Could you check a few things on this model? Use its own coordinates, in mm. Face numbers are marked on the shaded views. A direction names the side the tool comes from. Give positions to 0.01 mm unless a question says otherwise; leave off trailing zeros. Write each loop counter-clockwise with the first axis right and the second up, starting at its lowest first coordinate (ties: lowest second). Pieces come first, ordered by that corner, then holes. Notation, with made-up numbers: (-30.75, -8) - (21.25, -8) arc R18 ccw to (21.25, 18) - close; hole circle Ø8 at (-15.5, -27.5). An arc over 180 degrees is marked (long way). Answer in a Markdown table with one row per item.
from build123d import *

# Parameters (mm, degrees)
SKETCH1_R           = 7.338508892
SKETCH1_W           = 14.683745891
SKETCH1_H           = 15.594449323
BOSS_EXTRUDE6_DEPTH = 7.62


with BuildPart() as part:
    # Sketch1 → Boss-Extrude6 (new body)
    with BuildSketch(Plane(origin=(0, 0, 0), x_dir=(1, 0, 0), z_dir=(0, 1, 0))):
        with BuildLine():
            Line((-33.85382456, 51.361208868), (6.15117544, 51.361208868))
            ThreePointArc((6.15117544, 51.361208868), (9.743277889, 49.873311317), (11.23117544, 46.281208868))
            Line((11.23117544, 46.281208868), (11.23117544, 16.055208868))
            ThreePointArc((11.23117544, 16.055208868), (9.743277889, 12.46310642), (6.15117544, 10.975208868))
            Line((6.15117544, 10.975208868), (-33.85382456, 10.975208868))
            ThreePointArc((-33.85382456, 10.975208868), (-37.445927008, 12.46310642), (-38.93382456, 16.055208868))
            Line((-38.93382456, 16.055208868), (-38.93382456, 46.281208868))
            ThreePointArc((-38.93382456, 46.281208868), (-37.445927008, 49.873311317), (-33.85382456, 51.361208868))
        make_face()
        with Locations((-26.728784531, 42.288093859)):
            Circle(SKETCH1_R, mode=Mode.SUBTRACT)
        Polygon((-26.110126673, 13.007611736), (-27.479198511, 18.629319113), (-33.847743068, 18.629319113), (-28.993277919, 22.103725346), (-30.892236597, 27.725432723), (-26.110126673, 24.705324634), (-21.328016749, 27.725432723), (-23.076426813, 22.103725346), (-18.372510278, 18.629319113), (-24.17123819, 18.974896902), align=None, mode=Mode.SUBTRACT)
        with Locations((-1.086674016, 42.41081801)):
            Rectangle(SKETCH1_W, SKETCH1_H, mode=Mode.SUBTRACT)
        Polygon((5.867569864, 19.665294437), (-7.758291576, 27.532189206), (-7.758291576, 11.798399667), align=None, mode=Mode.SUBTRACT)
    extrude(amount=BOSS_EXTRUDE6_DEPTH)


solid = part.part
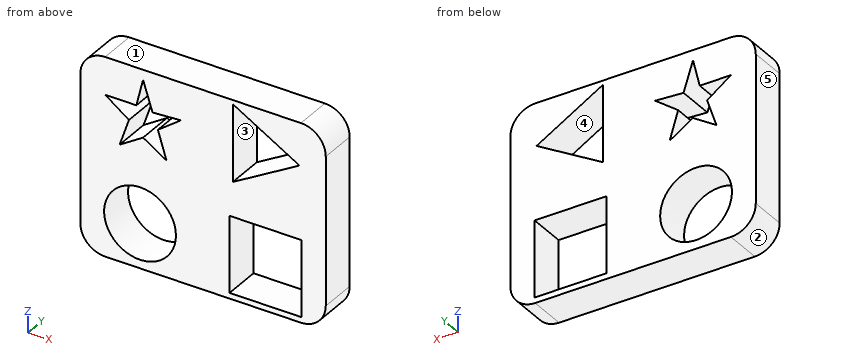
1) Imagine slicing it at D-D (x = 8). List the corners of the cut face in (y, z) for me, then the cut area to 3 significant figures.
Check values:
| item | result |
|---|---|
| outline | (0, -51.01) - (7.62, -51.01) - (7.62, -11.32) - (0, -11.32) - close |
| area | 302 mm2 |
2) Imagine slicing it at B-B (x = 2). List the corners of the cut face in (y, z) for me.
Check values:
| item | result |
|---|---|
| outline | (0, -51.36) - (7.62, -51.36) - (7.62, -50.21) - (0, -50.21) - close; (0, -34.61) - (7.62, -34.61) - (7.62, -21.9) - (0, -21.9) - close; (0, -17.43) - (7.62, -17.43) - (7.62, -10.98) - (0, -10.98) - close |
3) On a 3-axis mill with a long thin cutter (end or side, diameter ignored), from which of +Z, -Z, +X, -X, +Y, -Y can I reach the whole of each face in a straight line? I mean the marked faces 4 and 5. Say none if no direction works.
Check values:
| item | result |
|---|---|
| face 4 | +Y, -Y |
| face 5 | +Z, -Z, -X, +Y, -Y |
4) If I drill on line 1 (X direction, y = 5.75, z = -42.5); line 2 (Z direction, x = -7.5, y = 2.75); line 3 (X direction, y = 3.5, z = -35.5), over which ranges is the centre line in solid material (lowest first)?
Check values:
| item | result |
|---|---|
| line 1 | x = -38.93 to -34.06, -19.39 to -8.43, 6.26 to 11.23 |
| line 2 | z = -51.36 to -50.21, -34.61 to -27.38, -11.95 to -10.98 |
| line 3 | x = -38.93 to -29.52, -23.94 to -8.43, 6.26 to 11.23 |
5) We'd pull the mould along X, two halves only. Please class the marked faces 1, 2 and 3: +X half, -X half, draft (parallel to the pull), parting line (faces both ways), or undercut.
Check values:
| item | result |
|---|---|
| face 1 | draft |
| face 2 | -X half |
| face 3 | undercut |
6) Imagine slicing it at A-A (z = -17.5). List the corners of the cut face in (x, y) for me, then the cut area to 3 significant figures.
Check values:
| item | result |
|---|---|
| outline | (-38.93, 0) - (-27.2, 0) - (-27.2, 7.62) - (-38.93, 7.62) - close; (-24.65, 0) - (-7.76, 0) - (-7.76, 7.62) - (-24.65, 7.62) - close; (2.12, 0) - (11.23, 0) - (11.23, 7.62) - (2.12, 7.62) - close |
| area | 288 mm2 |
7) Imagine slicing it at C-C (y = 3.5). List the corners of the cut face in (x, z) for me.
Check values:
| item | result |
|---|---|
| outline | (-38.93, -46.28) arc R5.08 ccw to (-33.85, -51.36) - (6.15, -51.36) arc R5.08 ccw to (11.23, -46.28) - (11.23, -16.06) arc R5.08 ccw to (6.15, -10.98) - (-33.85, -10.98) arc R5.08 ccw to (-38.93, -16.06) - close; hole circle Ø14.68 at (-26.73, -42.29); hole (-33.85, -18.63) - (-28.99, -22.1) - (-30.89, -27.73) - (-26.11, -24.71) - (-21.33, -27.73) - (-23.08, -22.1) - (-18.37, -18.63) - (-24.17, -18.97) - (-26.11, -13.01) - (-27.48, -18.63) - close; hole (-8.43, -50.21) - (6.26, -50.21) - (6.26, -34.61) - (-8.43, -34.61) - close; hole (-7.76, -27.53) - (5.87, -19.67) - (-7.76, -11.8) - close |
